```python
from build123d import *

# Parameters (mm, degrees)
F0_R     = 38
F0_R_2   = 35
F1_DEPTH = 200
F2_R     = 5
F3_DEPTH = 125


with BuildPart() as f1:
    # F0 (on Top) → F1 (new body)
    with BuildSketch(Plane.XY):
        Circle(F0_R)
        Circle(F0_R_2, mode=Mode.SUBTRACT)
    extrude(amount=F1_DEPTH)


with BuildPart() as f3:
    # F2 (on Front) → F3 (new body)
    with BuildSketch(Plane.XZ):
        with Locations((-62.210366, -16.730187)):
            Circle(F2_R)
    extrude(amount=F3_DEPTH)


with BuildPart() as f3_1:
    # F4: moved
    add(f3.part.moved(Location((62.21, 60.4497, 177.31))))


with BuildPart() as f1_1:
    add(f1.part)

    # F5: cut F3
    add(f3_1.part, mode=Mode.SUBTRACT)


solid = f1_1.part
```
Can you work these out from the model? Positions are in its coordinate system, mm. Give positions to 0.01 mm unless a question says otherwise; leave off trailing zeros. Loops run counter-clockwise (first coordinate to the right, second up) from the corner with the lowest first, then second, coordinate; pieces in that order, holes last. Notation, with made-up numbers: M 8.25,-10.5 L 57.25,-10.5 A26 ccw 57.25,19.5 Z; hole C 40,48.25 d3. An arc over 180 degrees is marked long. Use one line per item in the form item = value. Start each with the question number.
(1) Please list where these lines run through material, in increasing order: line 1 (Y direction, x = 0, z = 94.5); line 2 (Y direction, x = -20.5, z = 44).
(2) I want a section at C-C, the plane x = 0. Write out the boundary of the cut face in (y, z), and give its area (3 significant figures).
(3) I want a section at B-B, the plane x = -27. Write out the boundary of the cut face in (y, z), and give its area (3 significant figures).
(4) I want a section at A-A, the plane y = 0. Write out the boundary of the cut face in (x, z), and give its area (3 significant figures).
(5) I want a section at D-D, the plane z = 143. Write out the boundary of the cut face in (x, y).
(6) I'm going to push flat-ended pins straight in: P1, Ø3, axis at y = 3, z = 148.5, coming from the -X side; P2, Ø6, axis at y = -26, z = 68.5, coming from the +X side; P3, Ø10, axis at x = 17.5, z = 101.5, coming from the -Y side. Where does each tip first touch, or does it pass through?
(7) Thinking about a two-plate mould opening in X: for faces 1 (the cylindrical face through (-0.651, 36.344, 165.537)), 2 (the flat face through (17, -31, 200)), 3 (the cylindrical face through (17.535, -33.713, 98.6)), which applies, released by +X, released by -X, zero draft, split by the parting line, or undercut?
Worked out:
q1.line_1 = -38 to -35, 35 to 38
q1.line_2 = -32 to -28.37, 28.37 to 32
q2.outline = M -38,0 L -35,0 L -35,155.58 L -38,155.58 Z; M -38,165.58 L -35,165.58 L -35,200 L -38,200 Z; M 35,0 L 38,0 L 38,155.58 L 35,155.58 Z; M 35,165.58 L 38,165.58 L 38,200 L 35,200 Z
q2.area = 1,140 mm²
q3.outline = M -26.74,0 L -22.27,0 L -22.27,200 L -26.74,200 Z; M 22.27,0 L 26.74,0 L 26.74,200 L 22.27,200 Z
q3.area = 1,790 mm²
q4.outline = M -38,0 L -35,0 L -35,200 L -38,200 Z; M 35,0 L 38,0 L 38,200 L 35,200 Z
q4.area = 1,200 mm²
q5.outline = C 0,0 d76; hole C 0,0 d70
q6.P1 = -37.97
q6.P2 = 30.25
q6.P3 = -35.89
q7.face_1 = undercut
q7.face_2 = zero draft
q7.face_3 = split by the parting line
